The drawing under review shows one solid part. Ordinate dimensions are in mm from its lowest x, y, z. A direction names the side the tool comes from. Coordinates: 2 decimals unless noted, no trailing zeros. Order: outer loops, then holes, each group sorted by start corner. A loop starts at its lowest first (then second) coordinate and runs counter-clockwise, first axis right, second up. Notation, with made-up numbers: M 2.5,-2 L 57.5,-2 A25 ccw 57.5,31 Z; hole C -26,60 d6. An arc over 180 degrees is marked long. Answer as a JSON object with one key per item and string values.
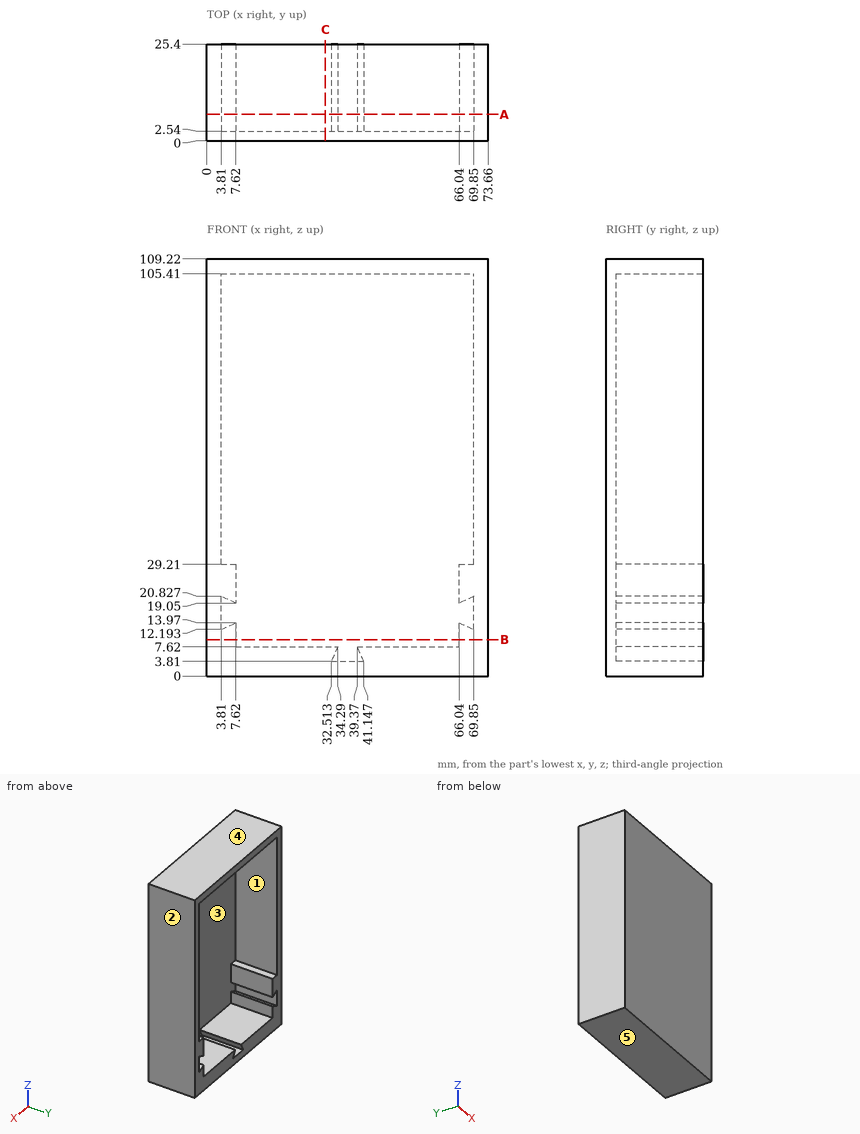
1) Mouldability with a two-part tool opening along Z and no side actions: class the marked faces 3, 4 and 5 as released by +Z, released by -Z, zero draft, split by the parting line, or undercut.
Taken from the geometry:
{"face 3": "undercut", "face 4": "released by +Z", "face 5": "released by -Z"}
2) Add section B-B (z = 9.5). State the section outline as (x, y) points.
Taken from the geometry:
{"outline": "M 0,0 L 73.66,0 L 73.66,25.4 L 66.04,25.4 L 66.04,2.54 L 7.62,2.54 L 7.62,25.4 L 0,25.4 Z"}
3) Tool access review of the marked faces 1 and 2: name each direction out of +Z, -Z, +X, -X, +Y, -Y from which nothing blocks a thin tool from reaching the whole face with its end or side.
Taken from the geometry:
{"face 1": "+Y", "face 2": "+Z, -Z, +X, +Y, -Y"}
4) Add section A-A (y = 7). State the section outline as (x, z) points.
Taken from the geometry:
{"outline": "M 0,0 L 73.66,0 L 73.66,109.22 L 0,109.22 Z; hole M 3.81,12.19 L 7.62,13.97 L 7.62,7.62 L 34.29,7.62 L 32.51,3.81 L 41.15,3.81 L 39.37,7.62 L 66.04,7.62 L 66.04,13.97 L 69.85,12.19 L 69.85,20.83 L 66.04,19.05 L 66.04,29.21 L 69.85,29.21 L 69.85,105.41 L 3.81,105.41 L 3.81,29.21 L 7.62,29.21 L 7.62,19.05 L 3.81,20.83 Z"}
5) Add section C-C (x = 31). State the section outline as (y, z) points.
Taken from the geometry:
{"outline": "M 0,0 L 25.4,0 L 25.4,7.62 L 2.54,7.62 L 2.54,105.41 L 25.4,105.41 L 25.4,109.22 L 0,109.22 Z"}
6) Insertion check: pin 1 Ø1.5 at (x, z) = (45, 37.5) entering from +Y. The pin has a flat end and moves straight along its axis. Give the tip position at first contact, or say it passes through.
Taken from the geometry:
{"pin 1": "stops at y = 2.54"}
7) To check wall thickness, follow L1, parallel to Z at x = 62, y = 17.5; L2, parallel to X at y = 8.75, z = 74; L3, parallel to Z at x = 68, y = 6.5 (1 decimal). State the ranges of each line that lie inside material, in increasing order.
Taken from the geometry:
{"L1": "z = 0 to 7.62, 105.41 to 109.22", "L2": "x = 0 to 3.81, 69.85 to 73.66", "L3": "z = 0 to 13.1, 20 to 29.2, 105.4 to 109.2"}
